Could you check a few things on this model? Use its own coordinates, in mm. A direction names the side the tool comes from. Round coordinates to 2 decimals unless told otherwise and drop trailing zeros. Write each loop counter-clockwise with the first axis right and the second up, starting at its lowest first coordinate (ties: lowest second). Pieces come first, ordered by that corner, then holes. Notation, with made-up numbers: (21, 58) -> (77, 58) arc R31 ccw to (77, 94) -> close; hole circle Ø11 at (71.5, 54). An arc over 180 degrees is marked (long way). Answer in a Markdown table with one row per item.
from build123d import *

# Parameters (mm, degrees)
SKETCH_1_W           = 45.4
SKETCH_1_H           = 27
EXTRUDE_1_DEPTH      = 7
SKETCH_2_R           = 1.6
CUT_EXTRUDE_1_DEPTH  = 62.727033531
SKETCH_4_R           = 3.1
EXTRUDE_2_DEPTH      = 5
SKETCH_5_W           = 45.4
SKETCH_5_H           = 12
EXTRUDE_3_DEPTH      = 20
SKETCH_7_R           = 5
CUT_EXTRUDE_3_DEPTH  = 6
EXTRUDE_4_DEPTH      = 14
SKETCH_10_W          = 8
SKETCH_10_H          = 12
CUT_EXTRUDE_6_DEPTH  = 2
SKETCH_12_R          = 2.2
CUT_EXTRUDE_8_DEPTH  = 6
SKETCH_13_R          = 2.2
CUT_EXTRUDE_9_DEPTH  = 6
SKETCH_14_W          = 45.4
SKETCH_14_H          = 24.5
SKETCH_14_R          = 3.1
EXTRUDE_5_DEPTH      = 52
SKETCH_15_W          = 12.5
SKETCH_15_H          = 36
CUT_EXTRUDE_10_DEPTH = 5
SKETCH_9_R           = 1.6
CUT_EXTRUDE_4_DEPTH  = 97.741548345
CUT_EXTRUDE_5_DEPTH  = 54.5
SKETCH_16_R          = 2.2
CUT_EXTRUDE_11_DEPTH = 6


with BuildPart() as part:
    # 草图1 → 凸台-拉伸1 (new body)
    with BuildSketch(Plane.XY):
        with Locations((-32.096319797, 14.04251269)):
            Rectangle(SKETCH_1_W, SKETCH_1_H)
    extrude(amount=EXTRUDE_1_DEPTH)

    # 草图2 → 切除-拉伸1 (cut, through all)
    with BuildSketch(Plane(origin=(0, 0, 0), x_dir=(-1, 0, 0), z_dir=(0, 0, -1))):
        with Locations((22.096319797, 24.04251269)):
            Circle(SKETCH_2_R)
        with Locations(Location((42.096319797, 24.04251269, 0), (0, 0, 180))):
            Circle(SKETCH_2_R)
        with Locations((42.096319797, 4.04251269)):
            Circle(SKETCH_2_R)
        with Locations(Location((22.096319797, 4.04251269, 0), (0, 0, 180))):
            Circle(SKETCH_2_R)
    extrude(amount=-CUT_EXTRUDE_1_DEPTH, mode=Mode.SUBTRACT)

    # 草图4 → 凸台-拉伸2 (add)
    with BuildSketch(Plane(origin=(0, 0, 0), x_dir=(-1, 0, 0), z_dir=(0, 0, -1))):
        Polygon((38.346319797, 0.54251269), (54.796319797, 0.54251269), (54.796319797, 27.54251269), (9.396319797, 27.54251269), (9.396319797, 0.54251269), (25.846319797, 0.54251269), align=None)
        with Locations(Location((42.096319797, 24.04251269, 0), (0, 0, 180))):
            Circle(SKETCH_4_R, mode=Mode.SUBTRACT)
        with Locations((22.096319797, 24.04251269)):
            Circle(SKETCH_4_R, mode=Mode.SUBTRACT)
        with Locations((42.096319797, 4.04251269)):
            Circle(SKETCH_4_R, mode=Mode.SUBTRACT)
        with Locations(Location((22.096319797, 4.04251269, 0), (0, 0, 180))):
            Circle(SKETCH_4_R, mode=Mode.SUBTRACT)
    extrude(amount=EXTRUDE_2_DEPTH)

    # 草图5 → 凸台-拉伸3 (add)
    with BuildSketch(Plane(origin=(0, 27.54251269, 0), x_dir=(1, 0, 0), z_dir=(0, 1, 0))):
        with Locations((-32.096319797, -1)):
            Rectangle(SKETCH_5_W, SKETCH_5_H)
    extrude(amount=EXTRUDE_3_DEPTH)

    # 草图7 → 切除-拉伸3 (cut)
    with BuildSketch(Plane(origin=(0, 0, -5), x_dir=(-1, 0, 0), z_dir=(0, 0, -1))):
        with BuildLine():
            Line((9.396319797, 38.14251269), (16.375464574, 38.14251269))
            ThreePointArc((16.375464574, 38.14251269), (18.004881648, 38.623584347), (19.111721141, 39.91251269))
            ThreePointArc((19.111721141, 39.91251269), (24.873653651, 44.014763896), (31.271319797, 40.998441785))
            ThreePointArc((31.271319797, 40.998441785), (32.096319797, 40.563574513), (32.921319797, 40.998441785))
            ThreePointArc((32.921319797, 40.998441785), (39.318985943, 44.014763896), (45.080918453, 39.91251269))
            ThreePointArc((45.080918453, 39.91251269), (46.187757946, 38.623584347), (47.81717502, 38.14251269))
            Line((47.81717502, 38.14251269), (54.796319797, 38.14251269))
            Line((54.796319797, 38.14251269), (54.796319797, 35.94251269))
            Line((54.796319797, 35.94251269), (47.81717502, 35.94251269))
            ThreePointArc((47.81717502, 35.94251269), (46.187757946, 35.461441034), (45.080918453, 34.17251269))
            ThreePointArc((45.080918453, 34.17251269), (39.318985943, 30.070261485), (32.921319797, 33.086583596))
            ThreePointArc((32.921319797, 33.086583596), (32.096319797, 33.521450868), (31.271319797, 33.086583596))
            ThreePointArc((31.271319797, 33.086583596), (24.873653651, 30.070261485), (19.111721141, 34.17251269))
            ThreePointArc((19.111721141, 34.17251269), (18.004881648, 35.461441034), (16.375464574, 35.94251269))
            Line((16.375464574, 35.94251269), (9.396319797, 35.94251269))
            Line((9.396319797, 35.94251269), (9.396319797, 38.14251269))
        make_face()
        with Locations((25.496319797, 37.04251269)):
            Circle(SKETCH_7_R, mode=Mode.SUBTRACT)
        with Locations(Location((38.696319797, 37.04251269, 0), (0, 0, 180))):
            Circle(SKETCH_7_R, mode=Mode.SUBTRACT)
    extrude(amount=-CUT_EXTRUDE_3_DEPTH, mode=Mode.SUBTRACT)

    # 草图8 → 凸台-拉伸4 (add)
    with BuildSketch(Plane.XZ.offset(-0.54251269)):
        Polygon((-54.796319797, 7), (-9.396319797, 7), (-9.396319797, -5), (-25.846319797, -5), (-38.346319797, -5), (-54.796319797, -5), align=None)
    extrude(amount=EXTRUDE_4_DEPTH)

    # 草图10 → 切除-拉伸6 (cut)
    with BuildSketch(Plane.XZ.offset(13.45748731)):
        with Locations((-45.796319797, 1)):
            Rectangle(SKETCH_10_W, SKETCH_10_H)
    extrude(amount=-CUT_EXTRUDE_6_DEPTH, mode=Mode.SUBTRACT)

    # 草图12 → 切除-拉伸8 (cut)
    with BuildSketch(Plane.XZ.offset(11.45748731)):
        with Locations(Location((-45.796319797, 1, 0), (0, 0, 270))):
            Circle(SKETCH_12_R)
    extrude(amount=-CUT_EXTRUDE_8_DEPTH, mode=Mode.SUBTRACT)

    # 草图13 → 切除-拉伸9 (cut)
    with BuildSketch(Plane(origin=(0, 0, -5), x_dir=(-1, 0, 0), z_dir=(0, 0, -1))):
        with Locations((32.096319797, 14.04251269)):
            Circle(SKETCH_13_R)
    extrude(amount=-CUT_EXTRUDE_9_DEPTH, mode=Mode.SUBTRACT)

    # 草图14 → 凸台-拉伸5 (add)
    with BuildSketch(Plane(origin=(0, 0, -5), x_dir=(-1, 0, 0), z_dir=(0, 0, -1))):
        with Locations((32.096319797, -1.20748731)):
            Rectangle(SKETCH_14_W, SKETCH_14_H)
        with Locations(Location((22.096319797, 4.04251269, 0), (0, 0, 180))):
            Circle(SKETCH_14_R, mode=Mode.SUBTRACT)
        with Locations((42.096319797, 4.04251269)):
            Circle(SKETCH_14_R, mode=Mode.SUBTRACT)
    extrude(amount=EXTRUDE_5_DEPTH)

    # 草图15 → 切除-拉伸10 (cut)
    with BuildSketch(Plane(origin=(0, 0, -57), x_dir=(-1, 0, 0), z_dir=(0, 0, -1))):
        with Locations((32.096319797, -13.45748731)):
            Rectangle(SKETCH_15_W, SKETCH_15_H)
    extrude(amount=-CUT_EXTRUDE_10_DEPTH, mode=Mode.SUBTRACT)

    # 草图9 → 切除-拉伸4 (cut, through all)
    with BuildSketch(Plane.XY.offset(7)):
        with Locations((-32.096319797, -8.95748731)):
            Circle(SKETCH_9_R)
    extrude(amount=-CUT_EXTRUDE_4_DEPTH, mode=Mode.SUBTRACT)

    # 草图3 → 切除-拉伸5 (cut)
    with BuildSketch(Plane.XY.offset(7)):
        Polygon((-28.920893316, -8.95748731), (-30.508606557, -6.20748731), (-33.684033037, -6.20748731), (-35.271746277, -8.95748731), (-33.684033037, -11.70748731), (-30.508606557, -11.70748731), align=None)
    extrude(amount=-CUT_EXTRUDE_5_DEPTH, mode=Mode.SUBTRACT)

    # 草图16 → 切除-拉伸11 (cut)
    with BuildSketch(Plane(origin=(0, 0, -57), x_dir=(-1, 0, 0), z_dir=(0, 0, -1))):
        with Locations((32.096319797, 8.04251269)):
            Circle(SKETCH_16_R)
    extrude(amount=-CUT_EXTRUDE_11_DEPTH, mode=Mode.SUBTRACT)


solid = part.part
1) Imagine slicing it at A-A, the plane y = -3. Please give me the cut outline in (x, z).
Findings:
| item | result |
|---|---|
| outline | (-54.8, -57) -> (-38.35, -57) -> (-38.35, -52) -> (-25.85, -52) -> (-25.85, -57) -> (-9.4, -57) -> (-9.4, 7) -> (-54.8, 7) -> close |
2) For pin 1 (3.5 mm diameter, centred on x = -45.8, z = 1, fed in from -Y); pin 2 (2 mm diameter, centred on x = -47, y = -13, fed in from +Z); pin 3 (4 mm diameter, centred on x = -42.5, z = -26.5, fed in from +Y); pin 4 (2.5 mm diameter, centred on x = -42.1, y = 4.04, fed in from -Z), each with a flat end and sliding along its axis, tell me the tip position at first contact or that it passes through.
Findings:
| item | result |
|---|---|
| pin 1 | stops at y = -5.46 |
| pin 2 | stops at z = -5 |
| pin 3 | stops at y = 11.04 |
| pin 4 | passes through |
3) Imagine slicing it at D-D, the plane z = -3.5. Count the separate pieces of the cut face and the enclosed holes in it, plus the area to 3 significant figures.
Findings:
| item | result |
|---|---|
| separate pieces | 4 |
| enclosed holes | 6 |
| area | 2,400 mm^2 |
4) Thinking about a two-plate mould opening in X: for faces 1 (the face through (-54.796, 3, -17)), 2 (the face through (-51, 35.943, -2)), 3 (the face through (-43.615, -8.499, 1.286)), which applies, +X half, -X half, draft (parallel to the pull), parting line (faces both ways), or undercut?
Findings:
| item | result |
|---|---|
| face 1 | -X half |
| face 2 | draft |
| face 3 | undercut |
5) Imagine slicing it at C-C, the plane x = -18. Please give me the cut outline in (y, z), plus the area to 3 significant figures.
Findings:
| item | result |
|---|---|
| outline | (-13.46, -57) -> (11.04, -57) -> (11.04, -5) -> (35.46, -5) -> (35.46, 1) -> (38.62, 1) -> (38.62, -5) -> (47.54, -5) -> (47.54, 7) -> (-13.46, 7) -> close |
| area | 1,990 mm^2 |
6) For faces 4 (the face through (-41.796, -12, 1)), 5 (the face through (-32, -11.707, -20)), 6 (the face through (-21.424, 21.016, -2.465)), which set-ups out of +Z, -Z, +X, -X, +Y, -Y let a thin tool reach every point of the face, with its end or its side?
Findings:
| item | result |
|---|---|
| face 4 | +Z, -Y |
| face 5 | +Z |
| face 6 | -Z |
7) Imagine slicing it at B-B, the plane z = -11.5. Please give me the cut outline in (x, y).
Findings:
| item | result |
|---|---|
| outline | (-54.8, -13.46) -> (-9.4, -13.46) -> (-9.4, 11.04) -> (-54.8, 11.04) -> close; hole circle Ø6.2 at (-42.1, 4.04); hole (-35.27, -8.96) -> (-33.68, -11.71) -> (-30.51, -11.71) -> (-28.92, -8.96) -> (-30.51, -6.21) -> (-33.68, -6.21) -> close; hole circle Ø6.2 at (-22.1, 4.04) |
8) Please list where these lines run through material, in increasing order: line 1 (Y direction, x = -37, z = -1); line 2 (Y direction, x = -47, z = -25); line 3 (Z direction, x = -20, y = 36).
Findings:
| item | result |
|---|---|
| line 1 | y = -13.46 to 30.25, 32.34 to 41.75, 43.83 to 47.54 |
| line 2 | y = -13.46 to 11.04 |
| line 3 | z = 1 to 7 |
